Part model, mm, in its own coordinate system. A direction names the side the tool comes from. Coordinates: 2 decimals unless noted, no trailing zeros. One line per question, with ' | ' between items. Start each with the question number.
1) Drop flat-ended pins along their axis: pin 1 (2.5 mm diameter, centred on x = -111.5, y = 16.5, fed in from +Z); pin 2 (4 mm diameter, centred on x = -34.75, y = 17.5, fed in from +Z); pin 3 (6.5 mm diameter, centred on x = 109.75, y = 7.5, fed in from -Z); pin 4 (1 mm diameter, centred on y = 9, z = 5, fed in from -X). Give the stop position or say it passes through.
2) 3-axis set-ups, long thin cutter, end or side, ignore diameter. For faces 4 (the face through (108, 26.7, 4)), 5 (the face through (108, 16.7, 3)), 6 (the face through (11, 35, 4)): which of +Z, -Z, +X, -X, +Y, -Y reach the whole face in a straight line?
3) Two-plate mould, pull along Y, no slides. Class faces 1 (the face through (14, 18, 8)), 2 (the face through (106.055, 15.968, 5.535)), 3 (the face through (-127.246, 17.115, 4.056)): released by +Y, released by -Y, zero draft, split by the parting line, or undercut.
4) Cut at A-A (z = 5.5). Count the separate pieces of the cut face and the enclosed holes in it, plus the area to 3 significant figures.
5) Probe L1, parallel to X at y = 21, z = 4.25; L2, parallel to X at y = 11, z = 1.5; L3, parallel to Y at x = -111.5, z = 6.5. List the from-to ranges inside material, lowest first. Write a range as from..to.
from build123d import *

# Parameters (mm, degrees)
CUT_EXTRUDE1_START         = -8.000000119
CUT_EXTRUDE1_OUTLINE_R     = 3.999999708
CUT_EXTRUDE1_OUTLINE_R_2   = 4
CUT_EXTRUDE1_OUTLINE_R_3   = 4.000000498
CUT_EXTRUDE1_OUTLINE_R_4   = 1.7
CUT_EXTRUDE1_DEPTH         = 8.000000119
CUT_EXTRUDE1_2_OUTLINE_R   = 4
CUT_EXTRUDE1_2_OUTLINE_R_2 = 1.7
CUT_EXTRUDE1_2_DEPTH       = 4.000000119
CUT_EXTRUDE1_START_2       = -3.000000119
CUT_EXTRUDE1_3_OUTLINE_R   = 4.000000498
CUT_EXTRUDE1_3_OUTLINE_R_2 = 1.699999454
CUT_EXTRUDE1_3_OUTLINE_R_3 = 3.999999708
CUT_EXTRUDE1_3_OUTLINE_R_4 = 1.700000883
CUT_EXTRUDE1_3_DEPTH       = 3.000000119
SKETCH2_R                  = 1.7
CUT_EXTRUDE2_DEPTH         = 133.217863668
BOSS_EXTRUDE1_START        = -8.000000119
BOSS_EXTRUDE1_DEPTH        = 8.000000119
SKETCH4_R                  = 4
SKETCH4_R_2                = 1.7
CUT_EXTRUDE3_DEPTH         = 4
SKETCH5_R                  = 1.7
CUT_EXTRUDE4_DEPTH         = 157.425904707


with BuildPart() as part:
    # Cut-Extrude1: read off the stored shape, not the designer's step
    # Cut-Extrude1 outline → Cut-Extrude1 (new body)
    # profile 1 of 3: a face of its own
    with BuildSketch(Plane(origin=(0, 0, 0), x_dir=(-1, 0, 0), z_dir=(0, 0, -1)).offset(CUT_EXTRUDE1_START)):
        with BuildLine():
            ThreePointArc((109.750003815, 0), (127.250003815, 17.5), (109.750003815, 35))
            Line((109.750003815, 35), (-109.750003815, 35))
            ThreePointArc((-109.750003815, 35), (-127.250003815, 17.5), (-109.750003815, 0))
            Line((-109.750003815, 0), (109.750003815, 0))
        make_face()
        with Locations((-109.750001685, 17.500000345)):
            Circle(CUT_EXTRUDE1_OUTLINE_R, mode=Mode.SUBTRACT)
        with Locations((-90.249998482, 17.5)):
            Circle(CUT_EXTRUDE1_OUTLINE_R_2, mode=Mode.SUBTRACT)
        with Locations((-3.249998482, 17.5)):
            Circle(CUT_EXTRUDE1_OUTLINE_R_2, mode=Mode.SUBTRACT)
        with Locations((34.750001518, 17.5)):
            Circle(CUT_EXTRUDE1_OUTLINE_R_2, mode=Mode.SUBTRACT)
        with Locations((97.750001518, 17.5)):
            Circle(CUT_EXTRUDE1_OUTLINE_R_2, mode=Mode.SUBTRACT)
        with Locations((109.750001518, 17.500000345)):
            Circle(CUT_EXTRUDE1_OUTLINE_R_3, mode=Mode.SUBTRACT)
    # profile 2 of 3: a face of its own
    with BuildSketch(Plane(origin=(0, 0, 0), x_dir=(-1, 0, 0), z_dir=(0, 0, -1)).offset(CUT_EXTRUDE1_START)):
        with Locations((-3.249998482, 17.5)):
            Circle(CUT_EXTRUDE1_OUTLINE_R_4)
    # profile 3 of 3: a face of its own
    with BuildSketch(Plane(origin=(0, 0, 0), x_dir=(-1, 0, 0), z_dir=(0, 0, -1)).offset(CUT_EXTRUDE1_START)):
        with Locations((-90.249998482, 17.5)):
            Circle(CUT_EXTRUDE1_OUTLINE_R_4)
    extrude(amount=CUT_EXTRUDE1_DEPTH)

    # Cut-Extrude1 2 outline → Cut-Extrude1 2 (add)
    # profile 1 of 4: a face of its own
    with BuildSketch(Plane(origin=(0, 0, 0), x_dir=(-1, 0, 0), z_dir=(0, 0, -1)).offset(CUT_EXTRUDE1_START)):
        with Locations((34.750001518, 17.5)):
            Circle(CUT_EXTRUDE1_2_OUTLINE_R)
        with Locations((34.750001518, 17.5)):
            Circle(CUT_EXTRUDE1_2_OUTLINE_R_2, mode=Mode.SUBTRACT)
    # profile 2 of 4: a face of its own
    with BuildSketch(Plane(origin=(0, 0, 0), x_dir=(-1, 0, 0), z_dir=(0, 0, -1)).offset(CUT_EXTRUDE1_START)):
        with Locations((97.750001518, 17.5)):
            Circle(CUT_EXTRUDE1_2_OUTLINE_R)
        with Locations((97.750001518, 17.5)):
            Circle(CUT_EXTRUDE1_2_OUTLINE_R_2, mode=Mode.SUBTRACT)
    # profile 3 of 4: a face of its own
    with BuildSketch(Plane(origin=(0, 0, 0), x_dir=(-1, 0, 0), z_dir=(0, 0, -1)).offset(CUT_EXTRUDE1_START)):
        with Locations((-3.249998482, 17.5)):
            Circle(CUT_EXTRUDE1_2_OUTLINE_R)
        with Locations((-3.249998482, 17.5)):
            Circle(CUT_EXTRUDE1_2_OUTLINE_R_2, mode=Mode.SUBTRACT)
    # profile 4 of 4: a face of its own
    with BuildSketch(Plane(origin=(0, 0, 0), x_dir=(-1, 0, 0), z_dir=(0, 0, -1)).offset(CUT_EXTRUDE1_START)):
        with Locations((-90.249998482, 17.5)):
            Circle(CUT_EXTRUDE1_2_OUTLINE_R)
        with Locations((-90.249998482, 17.5)):
            Circle(CUT_EXTRUDE1_2_OUTLINE_R_2, mode=Mode.SUBTRACT)
    extrude(amount=CUT_EXTRUDE1_2_DEPTH)

    # Cut-Extrude1 3 outline → Cut-Extrude1 3 (add)
    # profile 1 of 2: a face of its own
    with BuildSketch(Plane(origin=(0, 0, 0), x_dir=(-1, 0, 0), z_dir=(0, 0, -1)).offset(CUT_EXTRUDE1_START_2)):
        with Locations((109.750001518, 17.500000345)):
            Circle(CUT_EXTRUDE1_3_OUTLINE_R)
        with Locations((109.750002847, 17.500000345)):
            Circle(CUT_EXTRUDE1_3_OUTLINE_R_2, mode=Mode.SUBTRACT)
    # profile 2 of 2: a face of its own
    with BuildSketch(Plane(origin=(0, 0, 0), x_dir=(-1, 0, 0), z_dir=(0, 0, -1)).offset(CUT_EXTRUDE1_START_2)):
        with Locations((-109.750001685, 17.500000345)):
            Circle(CUT_EXTRUDE1_3_OUTLINE_R_3)
        with Locations((-109.750001213, 17.500000345)):
            Circle(CUT_EXTRUDE1_3_OUTLINE_R_4, mode=Mode.SUBTRACT)
    extrude(amount=CUT_EXTRUDE1_3_DEPTH)

    # Sketch2 → Cut-Extrude2 (cut, through all)
    with BuildSketch(Plane(origin=(0, 0, 0), x_dir=(-1, 0, 0), z_dir=(0, 0, -1))):
        with Locations((-90.249998482, 17.5)):
            Circle(SKETCH2_R)
        with Locations((-3.249998482, 17.5)):
            Circle(SKETCH2_R)
    extrude(amount=-CUT_EXTRUDE2_DEPTH, mode=Mode.SUBTRACT)

    # Sketch3 → Boss-Extrude1 (add)
    with BuildSketch(Plane(origin=(0, 0, 0), x_dir=(-1, 0, 0), z_dir=(0, 0, -1)).offset(BOSS_EXTRUDE1_START)):
        with BuildLine():
            Line((-109.750003815, 35), (-134.750003815, 35))
            ThreePointArc((-134.750003815, 35), (-152.250003815, 17.5), (-134.750003815, 0))
            Line((-134.750003815, 0), (-109.750003815, 0))
            ThreePointArc((-109.750003815, 0), (-127.250003815, 17.5), (-109.750003815, 35))
        make_face()
    extrude(amount=BOSS_EXTRUDE1_DEPTH)

    # Sketch4 → Cut-Extrude3 (cut)
    # profile 1 of 2: a face of its own
    with BuildSketch(Plane(origin=(0, 0, 0), x_dir=(-1, 0, 0), z_dir=(0, 0, -1))):
        with Locations((-109.750001213, 27.500000345)):
            Circle(SKETCH4_R)
        with Locations((-109.750001213, 27.500000345)):
            Circle(SKETCH4_R_2, mode=Mode.SUBTRACT)
    # profile 2 of 2: a face of its own
    with BuildSketch(Plane(origin=(0, 0, 0), x_dir=(-1, 0, 0), z_dir=(0, 0, -1))):
        with Locations(Location((-109.750001213, 7.500000345, 0), (0, 0, 180))):
            Circle(SKETCH4_R)
        with Locations(Location((-109.750001213, 7.500000345, 0), (0, 0, 180))):
            Circle(SKETCH4_R_2, mode=Mode.SUBTRACT)
    extrude(amount=-CUT_EXTRUDE3_DEPTH, mode=Mode.SUBTRACT)

    # Sketch5 → Cut-Extrude4 (cut, through all)
    with BuildSketch(Plane(origin=(0, 0, 0), x_dir=(-1, 0, 0), z_dir=(0, 0, -1))):
        with Locations((-109.750001213, 27.500000345)):
            Circle(SKETCH5_R)
        with Locations((-109.750001213, 7.500000345)):
            Circle(SKETCH5_R)
    extrude(amount=-CUT_EXTRUDE4_DEPTH, mode=Mode.SUBTRACT)


solid = part.part
Reported:
1) pin 1: stops at z = 3 | pin 2: stops at z = 8 | pin 3: stops at z = 4 | pin 4: stops at x = -125.31
2) face 4: -Z | face 5: +Z | face 6: +Z, -Z, +X, -X, +Y
3) face 1: zero draft | face 2: undercut | face 3: split by the parting line
4) separate pieces: 1 | enclosed holes: 8 | area: 9,360 mm²
5) L1: x = -126.9..-111.69, -107.81..107.81, 111.69..151.9 | L2: x = -126..107.81, 111.69..151 | L3: y = 0.09..13.9, 21.1..34.91
